For this review, take the finished solid that the model builds, in its own axes (mm). Face numbers are marked on the shaded views. A direction names the side the tool comes from. Round coordinates to 2 decimals unless told otherwise and drop trailing zeros. Order: outer loops, then holes, each group sorted by start corner. A loop starts at its lowest first (then second) coordinate and runs counter-clockwise, first axis right, second up.
from build123d import *

# Parameters (mm, degrees)
BOSS_EXTRUDE1_DEPTH = 5.6134
CIRPATTERN1_COUNT   = 12


# Read off the part's stored shape, not the designer's step: ThreadSchematic
with BuildPart() as part:
    # ThreadSchematic outline → ThreadSchematic (revolve)
    with BuildSketch(Plane.YX):
        with BuildLine():
            Line((0, 16.9164), (0, 0))
            ThreePointArc((0, 0), (4.915818779, 1.070865158), (8.940800003, 4.089400003))
            Line((8.940800003, 4.089400003), (8.9408, 4.2164))
            Line((8.9408, 4.2164), (4.75615, 4.2164))
            ThreePointArc((4.75615, 4.2164), (4.19937412, 4.44702412), (3.96875, 5.0038))
            Line((3.96875, 5.0038), (3.96875, 16.9164))
            Line((3.96875, 16.9164), (0, 16.9164))
        make_face()
    revolve(axis=Axis((0, 0, 0), (1, 0, 0)))

    # Sketch2 → Boss-Extrude1 (add)
    with BuildSketch(Plane(origin=(5.3594, 0, 0), x_dir=(0, 0, -1), z_dir=(1, 0, 0))):
        Polygon((-4.318, 0), (-3.95182104, -0.36617896), (0, 0), (-3.95182104, 0.36617896), align=None)
    boss_extrude1 = extrude(amount=BOSS_EXTRUDE1_DEPTH)

    # CirPattern1: Boss-Extrude1 ×12 about axis
    cirpattern1_axis = Axis((0, 0, 0), (1, 0, 0))
    for i in range(1, CIRPATTERN1_COUNT):
        add(boss_extrude1.rotate(cirpattern1_axis, i * 360 / CIRPATTERN1_COUNT))


solid = part.part
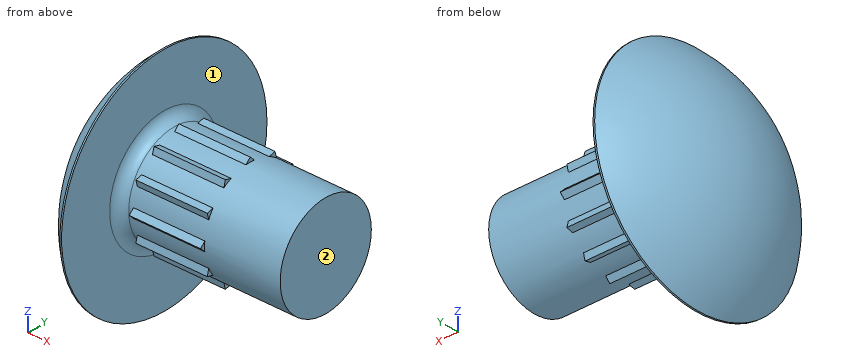
(1) Add section A-A on x = 11.25. Give the boundary of the cut face in (y, z).
(2) Clearance check with flat-ended pins moving along their axes: P1, Ø5, axis at x = 3.5, z = 5, coming from the -Y side; P2, Ø10, axis at x = 9, y = -0.5, coming from the -Z side; P3, Ø3, axis at x = 13, y = 3, coming from the +Z side; P4, Ø1, axis at y = -2, z = 2, coming from the -X side. State where each tip first meets the part, or that it passes through.
(3) Wall thickness on L1, parallel to Y at x = 3, z = 1; L2, parallel to X at y = 2, z = 5.5; L3, parallel to Z at x = 3.75, y = 0.75: over which ranges is each line inside the solid? List them lowest first.
(4) Add section B-B on z = 7.25. Give the boundary of the cut face in (x, y).
(5) Tool access review of the marked faces 1 and 2: name each direction out of +Z, -Z, +X, -X, +Y, -Y from which nothing blocks a thin tool from reaching the whole face with its end or side.
Here are the results:
1. outline: circle Ø7.94 at (0, 0)
2. P1: stops at y = -8.56
2. P2: stops at z = -8.94
2. P3: stops at z = 3.67
2. P4: stops at x = 0.23
3. L1: y = -7.8 to 7.8
3. L2: x = 1.55 to 4.22
3. L3: z = -8.6 to 8.6
4. outline: (4.09, -5.23) - (4.22, -5.23) - (4.22, 5.23) - (4.09, 5.23) arc R9.33 ccw to start
5. face 1: +X
5. face 2: +Z, -Z, +X, +Y, -Y
